Design review of the part shown in the three views and the two pictorial views. Dimensions are in mm from the part's minimum x, y and z. A direction names the side the tool comes from. Give positions to 0.01 mm unless a question says otherwise; leave off trailing zeros. Loops run counter-clockwise (first coordinate to the right, second up) from the corner with the lowest first, then second, coordinate; pieces in that order, holes last. Notation, with made-up numbers: (-8.75, -26) - (-4.75, -26) arc R33 cw to (-4.75, 4) - close; hole circle Ø10 at (-3.5, -17.5). An arc over 180 degrees is marked (long way). Use CSV: the item, a comma, the result in double quotes. Start each with the question number.
1. Take a section at A-A on x = 3.25. Give the boundary of the cut face in (y, z), plus the area to 3 significant figures.
2. For the marked faces 1, 2 and 3, list the 3-axis set-ups (+Z, -Z, +X, -X, +Y, -Y) from which the entire face can be reached by the end or side of a thin tool; tool diameter is ignored.
3. Take a section at B-B on y = 11.5. Give the boundary of the cut face in (x, z).
4. For pin 1 (5 mm diameter, centred on y = 6.5, z = 12.5, fed in from -X); pin 2 (1.5 mm diameter, centred on y = 9, z = 17, fed in from -X); pin 3 (0.5 mm diameter, centred on x = 9, z = 12.5, fed in from +Y), all flat-tipped, find the tip position at first contact; note any pin that passes through.
5. Mouldability with a two-part tool opening along Z and no side actions: class the marked faces 4, 5, 6 and 7 as pulls with the +Z half, pulls with the -Z half, needs draft (parallel to the pull), parting line crosses it, or undercut.
6. Take a section at D-D on z = 7.25. Give the boundary of the cut face in (x, y), plus the area to 3 significant figures.
7. Wall thickness on line 1 (X direction, y = 6, z = 17); line 2 (X direction, y = 3, z = 12.25); line 3 (Z direction, x = 2.5, y = 9): over which ranges is each line inside the solid? List them lowest first.
8. Take a section at C-C on z = 2. Give the boundary of the cut face in (x, y), plus the area to 3 significant figures.
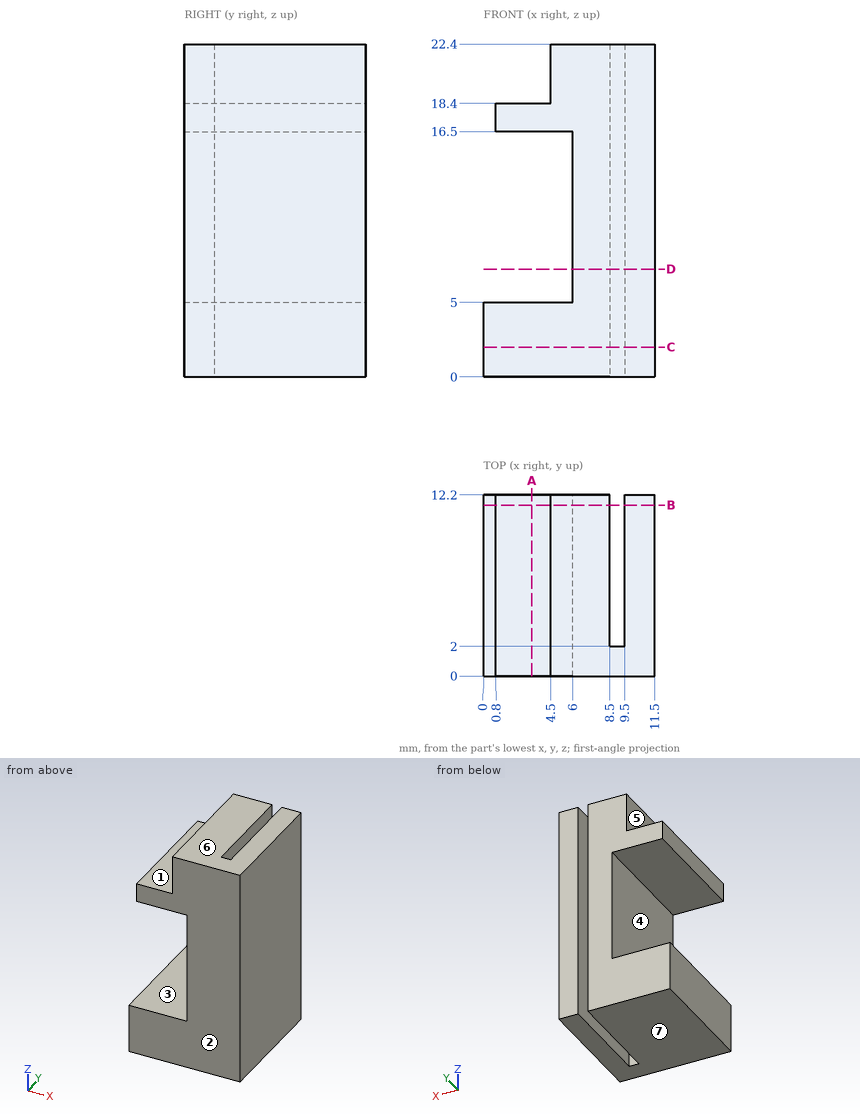
Check result:
1,outline,"(0, 0) - (12.2, 0) - (12.2, 5) - (0, 5) - close; (0, 16.5) - (12.2, 16.5) - (12.2, 18.4) - (0, 18.4) - close"
1,area,"84.2 mm²"
2,face 1,"+Z, -X, +Y, -Y"
2,face 2,"+Z, -Z, +X, -X, -Y"
2,face 3,"-X, +Y, -Y"
3,outline,"(0, 0) - (8.5, 0) - (8.5, 22.4) - (4.5, 22.4) - (4.5, 18.4) - (0.8, 18.4) - (0.8, 16.5) - (6, 16.5) - (6, 5) - (0, 5) - close; (9.5, 0) - (11.5, 0) - (11.5, 22.4) - (9.5, 22.4) - close"
4,pin 1,"stops at x = 6"
4,pin 2,"stops at x = 0.8"
4,pin 3,"stops at y = 2"
5,face 4,"undercut"
5,face 5,"needs draft"
5,face 6,"pulls with the +Z half"
5,face 7,"pulls with the -Z half"
6,outline,"(6, 0) - (11.5, 0) - (11.5, 12.2) - (9.5, 12.2) - (9.5, 2) - (8.5, 2) - (8.5, 12.2) - (6, 12.2) - close"
6,area,"56.9 mm²"
7,line 1,"x = 0.8 to 8.5, 9.5 to 11.5"
7,line 2,"x = 6 to 8.5, 9.5 to 11.5"
7,line 3,"z = 0 to 5, 16.5 to 18.4"
8,outline,"(0, 0) - (11.5, 0) - (11.5, 12.2) - (9.5, 12.2) - (9.5, 2) - (8.5, 2) - (8.5, 12.2) - (0, 12.2) - close"
8,area,"130 mm²"
